Here's how the part is built. I have some questions about the finished solid (model axes, mm). Face numbers are marked on the shaded views. Coordinates: 2 decimals unless noted, no trailing zeros. Write each loop counter-clockwise with the first axis right and the second up, starting at its lowest first coordinate (ties: lowest second). Pieces come first, ordered by that corner, then holes. Notation, with made-up numbers: (-33, 22.25) - (21, 22.25) arc R19 ccw to (21, 48.25) - close; hole circle Ø11 at (-21, 36.5). An arc over 180 degrees is marked (long way). Answer in a Markdown table with one row per item. Add a question column.
Item 1: Imagine slicing it at D-D (x = -155). Please give me the cut outline in (y, z), plus the area to 3 significant figures.
Item 2: If I drill on probe 1 along Y at (x, z) = (-238.5, 8.75); probe 2 along X at (y, z) = (-130, 9.25); probe 3 along X at (y, z) = (64, 3), over which ranges is the centre line in solid material (lowest first)? Write a range as from..to.
Item 3: I'm going to push flat-ended pins straight in: pin 1 (10.5 mm diameter, centred on x = -487.5, y = -130, fed in from -Z); pin 2 (10 mm diameter, centred on y = -84, z = 2.5, fed in from +X); pin 3 (3.5 mm diameter, centred on x = -240, y = -130.5, fed in from +Z); pin 4 (2 mm diameter, centred on x = 53, z = 9, fed in from -Y). Where does each tip first touch, or does it pass through?
Item 4: Imagine slicing it at C-C (y = 103). Please give me the cut outline in (x, z), plus the area to 3 significant figures.
Item 5: We'd pull the mould along Y, two halves only. Please class the marked faces 1 and 2: +Y half, -Y half, draft (parallel to the pull), parting line (faces both ways), or undercut.
Item 6: Imagine slicing it at A-A (y = -9). Please give me the cut outline in (x, z).
Item 7: Imagine slicing it at B-B (x = -430). Please give me the cut outline in (y, z).
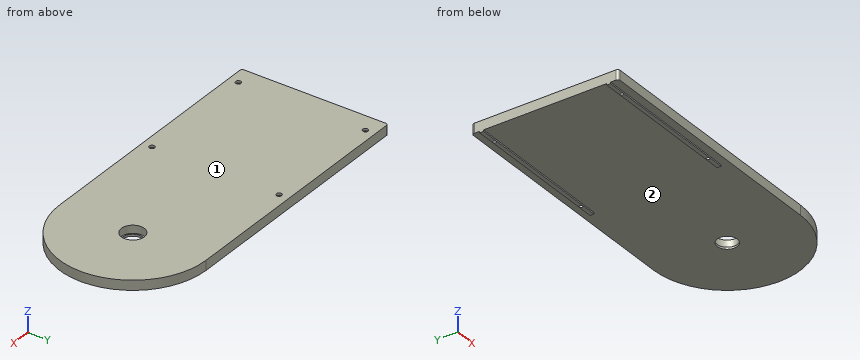
from build123d import *

# Parameters (mm, degrees)
SKETCH1_R           = 20.5
BOSS_EXTRUDE1_DEPTH = 20
SKETCH2_R           = 23.5
CUT_EXTRUDE1_DEPTH  = 16
SKETCH4_W           = 318.75
SKETCH4_H           = 8
BOSS_EXTRUDE2_DEPTH = 3
SKETCH3_R           = 3.25
CUT_EXTRUDE2_DEPTH  = 547.492451915
SKETCH5_R           = 5.5
CUT_EXTRUDE3_DEPTH  = 4.5
FILLET1_R           = 5


with BuildPart() as part:
    # Sketch1 → Boss-Extrude1 (new body)
    with BuildSketch(Plane.XY):
        with BuildLine():
            Line((0, 150), (-525, 150))
            Line((-525, 150), (-525, -150))
            Line((-525, -150), (0, -150))
            ThreePointArc((0, -150), (150, 0), (0, 150))
        make_face()
        Circle(SKETCH1_R, mode=Mode.SUBTRACT)
    extrude(amount=BOSS_EXTRUDE1_DEPTH)

    # Sketch2 → Cut-Extrude1 (cut)
    with BuildSketch(Plane.XY.offset(20)):
        Circle(SKETCH2_R)
    extrude(amount=-CUT_EXTRUDE1_DEPTH, mode=Mode.SUBTRACT)

    # Sketch4 → Boss-Extrude2 (add)
    with BuildSketch(Plane(origin=(0, 0, 0), x_dir=(-1, 0, 0), z_dir=(0, 0, -1))):
        with Locations((365.625, -130)):
            Rectangle(SKETCH4_W, SKETCH4_H)
        with Locations((365.625, 130)):
            Rectangle(SKETCH4_W, SKETCH4_H)
    extrude(amount=BOSS_EXTRUDE2_DEPTH)

    # Sketch3 → Cut-Extrude2 (cut, through all)
    with BuildSketch(Plane.XY.offset(20)):
        with Locations((-238.5, 130)):
            Circle(SKETCH3_R)
        with Locations((-487.5, 130)):
            Circle(SKETCH3_R)
        with Locations((-487.5, -130)):
            Circle(SKETCH3_R)
        with Locations((-238.5, -130)):
            Circle(SKETCH3_R)
    extrude(amount=-CUT_EXTRUDE2_DEPTH, mode=Mode.SUBTRACT)

    # Sketch5 → Cut-Extrude3 (cut)
    with BuildSketch(Plane.XY.offset(20)):
        with Locations((-487.5, 130)):
            Circle(SKETCH5_R)
        with Locations((-238.5, 130)):
            Circle(SKETCH5_R)
        with Locations((-238.5, -130)):
            Circle(SKETCH5_R)
        with Locations((-487.5, -130)):
            Circle(SKETCH5_R)
    extrude(amount=-CUT_EXTRUDE3_DEPTH, mode=Mode.SUBTRACT)

    # Fillet1
    fillet1_edges = [part.edges().sort_by_distance(p)[0] for p in [
        (-525, -150, 10),
        (-525, 150, 10),
    ]]
    fillet(fillet1_edges, radius=FILLET1_R)


solid = part.part
Here are the results:
| question | item | result |
|---|---|---|
| 1 | outline | (-150, 0) - (150, 0) - (150, 20) - (-150, 20) - close |
| 1 | area | 6,000 mm2 |
| 2 | probe 1 | y = -150..-133.25, -126.75..126.75, 133.25..150 |
| 2 | probe 2 | x = -525..-490.75, -484.25..-241.75, -235.25..74.83 |
| 2 | probe 3 | x = -525..135.66 |
| 3 | pin 1 | stops at z = -3 |
| 3 | pin 2 | stops at x = 127.51 |
| 3 | pin 3 | stops at z = 15.5 |
| 3 | pin 4 | stops at y = -140.7 |
| 4 | outline | (-525, 0) - (109.05, 0) - (109.05, 20) - (-525, 20) - close |
| 4 | area | 12,700 mm2 |
| 5 | face 1 | draft |
| 5 | face 2 | undercut |
| 6 | outline | (-525, 0) - (-18.42, 0) - (-18.42, 4) - (-21.71, 4) - (-21.71, 20) - (-525, 20) - close; (18.42, 0) - (149.73, 0) - (149.73, 20) - (21.71, 20) - (21.71, 4) - (18.42, 4) - close |
| 7 | outline | (-150, 0) - (-134, 0) - (-134, -3) - (-126, -3) - (-126, 0) - (126, 0) - (126, -3) - (134, -3) - (134, 0) - (150, 0) - (150, 20) - (-150, 20) - close |
